Can you work these out from the model? Positions are in its coordinate system, mm. Face numbers are marked on the shaded views. A direction names the side the tool comes from. Give positions to 0.01 mm unless a question says otherwise; leave off trailing zeros. Order: outer loops, then holes, each group sorted by start corner. A loop starts at its lowest first (then second) coordinate and runs counter-clockwise, first axis right, second up.
Autodesk Inventor part; units mm, degrees
ref_plane "YZ Plane" through (0, 0, 0) normal (1, 0, 0) x (0, 1, 0)
ref_plane "XZ Plane" through (0, 0, 0) normal (0, 1, 0) x (-1, 0, 0)
ref_plane "XY Plane" through (0, 0, 0) normal (0, 0, 1) x (1, 0, 0)
sketch "Sketch1" plane through (0, 0, 0) normal (0, 0, 1) x (1, 0, 0)
  line L0 (0, 14.375) -> (0, 5.6)
  line L1 (0, 14.375) -> (0, 17.5)
  line L2 (-0.35, 17.5) -> (-0.35, 15.554)
  line L3 (0, 17.5) -> (0, 5.6)
  line L4 (-0.35, 17.5) -> (0, 17.5)
  line L5 (-5, 7.5) -> (-0.35, 15.554)
  line L6 (-5, 7.5) -> (6.0041, 7.5) construction
  line L7 (-5, -2.5) -> (-2.8, -2.5)
  line L8 (-2.8, -2.5) -> (0, -2.5)
  line L9 (0, -2.5) -> (0, 5.6)
  line L10 (-5, 7.5) -> (-5, 5.5)
  line L11 (-5, 5.5) -> (-4.5, 5.5)
  line L12 (-4.5, 5.5) -> (-4.5, 3)
  line L13 (-4.5, 3) -> (-5, 3)
  line L14 (-5, 7.5) -> (-5, 5.5)
  line L15 (-5, 3) -> (-5, -2.5)
  dimension "d81" = 60
  dimension "d82" = 10
  dimension "d83" = 0.35
  dimension "d84" = 1.946
  dimension "d85" = 8.054
  dimension "d87" = 10
  dimension "d106" = 20
  dimension "d107" = 5
  dimension "d131" = 2
  dimension "d132" = 0.5
  dimension "d133" = 2.5
revolve "Revolution1" add sketch "Sketch1" angle 360 about axis through (0, 14.375, 0) along (0, -1, 0)
ref_plane "Work Plane3" through (0, -2.5, 0) normal (0, 1, 0) x (-1, 0, 0)
sketch "Sketch5" plane through (0, -2.5, 0) normal (0, 1, 0) x (-1, 0, 0)
  point P0 (0, 0)
sketch "Sketch6" plane through (0, -2.5, 0) normal (0, -1, 0) x (1, 0, 0)
  circle A0 centre (0, 0) radius 2.9
  dimension "d108" = 5.8
hole "Hole6" at (0, -2.5, 0) direction (0, 1, 0) diameter 5.8 depth 7.25 tip angle 118
hole "Hole7" at (0, -2.5, 0) direction (0, 1, 0) diameter 2 depth 15 tip angle 118
sketch "Sketch7" plane through (0, 17.5, 0) normal (0, 1, 0) x (1, 0, 0)
  circle A0 centre (0, 0) radius 0.075
  dimension "d123" = 0.15
hole "Hole8" at (0, 17.5, 0) direction (0, -1, 0) diameter 0.3 end through all
properties part number "Nozzle"
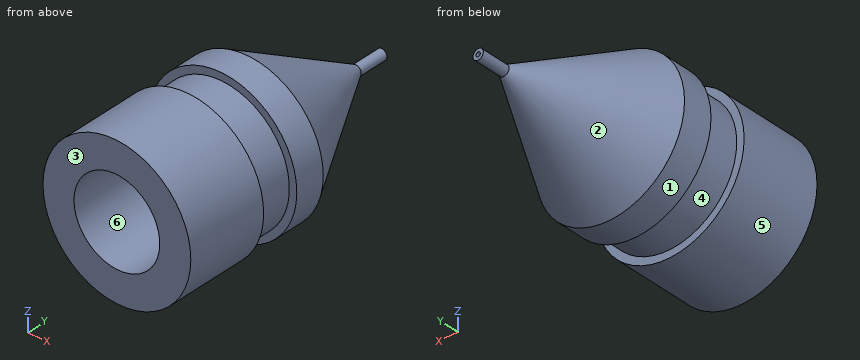
1) We'd pull the mould along Y, two halves only. Please class the marked faces 1, 2, 3 and 4: +Y half, -Y half, draft (parallel to the pull), parting line (faces both ways), or undercut.
2) Suppose I cut it at B-B (y = 0.25). Please give me the cut outline in (x, z).
3) Which directions (+Z, -Z, +X, -X, +Y, -Y) give clear straight access to the entire face, cutting with the end or side of a thin tool? Please do the marked faces 5 and 6.
4) I'm going to push flat-ended pins straight in: pin 1 Ø5 at (y, z) = (11.5, 1) entering from -X; pin 2 Ø4 at (x, z) = (-3, 4) entering from +Y; pin 3 Ø1.5 at (y, z) = (10.5, 2) entering from -X; pin 4 Ø3 at (y, z) = (1, 1.5) entering from -X. Where does each tip first touch, or does it pass through?
5) If I drill on line 1 (X direction, y = 15.75, z = 0); line 2 (X direction, y = 0.5, z = 0); line 3 (Z direction, x = -2.5, y = 1.75), over which ranges is the centre line in solid material (lowest first)?
6) Suppose I cut it at A-A (y = 14.5). Please give me the cut outline in (x, z), and give its area (3 significant figures).
Results:
1. face 1: draft
1. face 2: +Y half
1. face 3: -Y half
1. face 4: undercut
2. outline: circle Ø10 at (0, 0); hole circle Ø5.8 at (0, 0)
3. face 5: +Y, -Y
3. face 6: -Y
4. pin 1: stops at x = -4.07
4. pin 2: stops at y = 10.96
4. pin 3: stops at x = -3.27
4. pin 4: stops at x = -5
5. line 1: x = -0.35 to -0.15, 0.15 to 0.35
5. line 2: x = -5 to -2.9, 2.9 to 5
5. line 3: z = -4.33 to -1.47, 1.47 to 4.33
6. outline: circle Ø1.92 at (0, 0); hole circle Ø0.3 at (0, 0)
6. area: 2.82 mm2
